Could you check a few things on this model? Use its own coordinates, in mm. Round coordinates to 2 decimals unless told otherwise and drop trailing zeros. Loops run counter-clockwise (first coordinate to the right, second up) from the corner with the lowest first, then second, coordinate; pieces in that order, holes last. Notation, with made-up numbers: M 13,41 L 65,41 A19 ccw 65,67 Z; hole C 50.5,30.25 d6. An arc over 180 degrees is marked long. Answer in a Markdown table with one row per item.
```python
from build123d import *

# Parameters (mm, degrees)
CROQUIS1_W                 = 73.8
CROQUIS1_H                 = 73.8
SALIENTE_EXTRUIR3_DEPTH    = 1.9
CROQUIS2_R                 = 1.5
CORTAR_EXTRUIR1_DEPTH      = 1
CORTAR_EXTRUIR1_DEPTH_BACK = 2.9


with BuildPart() as part:
    # Croquis1 → Saliente-Extruir3 (new body)
    with BuildSketch(Plane(origin=(0, 0, 0), x_dir=(1, 0, 0), z_dir=(0, 1, 0))):
        Rectangle(CROQUIS1_W, CROQUIS1_H)
    extrude(amount=SALIENTE_EXTRUIR3_DEPTH)

    # Croquis2 → Cortar-Extruir1 (cut, two sides)
    with BuildSketch(Plane(origin=(0, 1.9, 0), x_dir=(1, 0, 0), z_dir=(0, 1, 0))) as cortar_extruir1_sk:
        with Locations((-28.9, 0)):
            Circle(CROQUIS2_R)
        with Locations((28.9, 0)):
            Circle(CROQUIS2_R)
    extrude(amount=CORTAR_EXTRUIR1_DEPTH, mode=Mode.SUBTRACT)
    extrude(cortar_extruir1_sk.sketch, amount=-CORTAR_EXTRUIR1_DEPTH_BACK, mode=Mode.SUBTRACT)


solid = part.part
```
1) I need wall thicknesses on line 1 (X direction, y = 1.2, z = 0); line 2 (Z direction, x = 28.9, y = 1.35); line 3 (Z direction, x = -28.5, y = 1.65). Which ranges of each line are inside material? Lowest first, please.
Computed:
| item | result |
|---|---|
| line 1 | x = -36.9 to -30.4, -27.4 to 27.4, 30.4 to 36.9 |
| line 2 | z = -36.9 to -1.5, 1.5 to 36.9 |
| line 3 | z = -36.9 to -1.45, 1.45 to 36.9 |
2) If we mould it in two halves opening along Z, with no side actions, what happens to faces 1 (the face through (-1, 1, -36.9)), 2 (the face through (-36.9, 1, 1)), 3 (the face through (-30.4, 0.96, -0.07))? For each: released by +Z, released by -Z, zero draft, split by the parting line, or undercut.
Computed:
| item | result |
|---|---|
| face 1 | released by -Z |
| face 2 | zero draft |
| face 3 | undercut |
3) I want a section at A-A, the plane x = -28.9. Please give me the cut outline in (y, z), plus the area to 3 significant figures.
Computed:
| item | result |
|---|---|
| outline | M 0,-36.9 L 1.9,-36.9 L 1.9,-1.5 L 0,-1.5 Z; M 0,1.5 L 1.9,1.5 L 1.9,36.9 L 0,36.9 Z |
| area | 135 mm² |
4) I want a section at B-B, the plane z = 0. Please give me the cut outline in (x, y), plus the area to 3 significant figures.
Computed:
| item | result |
|---|---|
| outline | M -36.9,0 L -30.4,0 L -30.4,1.9 L -36.9,1.9 Z; M -27.4,0 L 27.4,0 L 27.4,1.9 L -27.4,1.9 Z; M 30.4,0 L 36.9,0 L 36.9,1.9 L 30.4,1.9 Z |
| area | 129 mm² |
